Answer from the drawing. Dimensions are ordinates in mm from the lowest x, y and z of the part. Give positions to 0.01 mm unless a question says otherwise; leave off trailing zeros. Loops run counter-clockwise (first coordinate to the right, second up) from the corner with the lowest first, then second, coordinate; pieces in that order, holes last.
Item 1: Section C-C, the plane x = 26 is taken. Give the vertices of the cut face in (y, z) (1 decimal).
Item 2: This flat-tipped pin is pushed along its axis until it touches: pin 1 Ø0.8 at (y, z) = (1.5, 86.5) entering from -X. Where does it stop, or does it pass through?
Item 3: Section B-B, the plane z = 85.5 is taken. Give the vertices of the cut face in (x, y) (1 decimal).
Item 4: Consider line 1 along X through (y, z) = (0.5, 88.5) (1 decimal); line 2 along X through (y, z) = (1, 85) (1 decimal); line 3 along X through (y, z) = (1.95, 67). Determine where each line is inside the solid, lowest interval first.
Item 5: Section A-A, the plane y = 1.9 is taken. Give the vertices of the cut face in (x, z) (1 decimal).
Item 6: Section D-D, the plane z = 65 is taken. Give the vertices of the cut face in (x, y) (1 decimal).
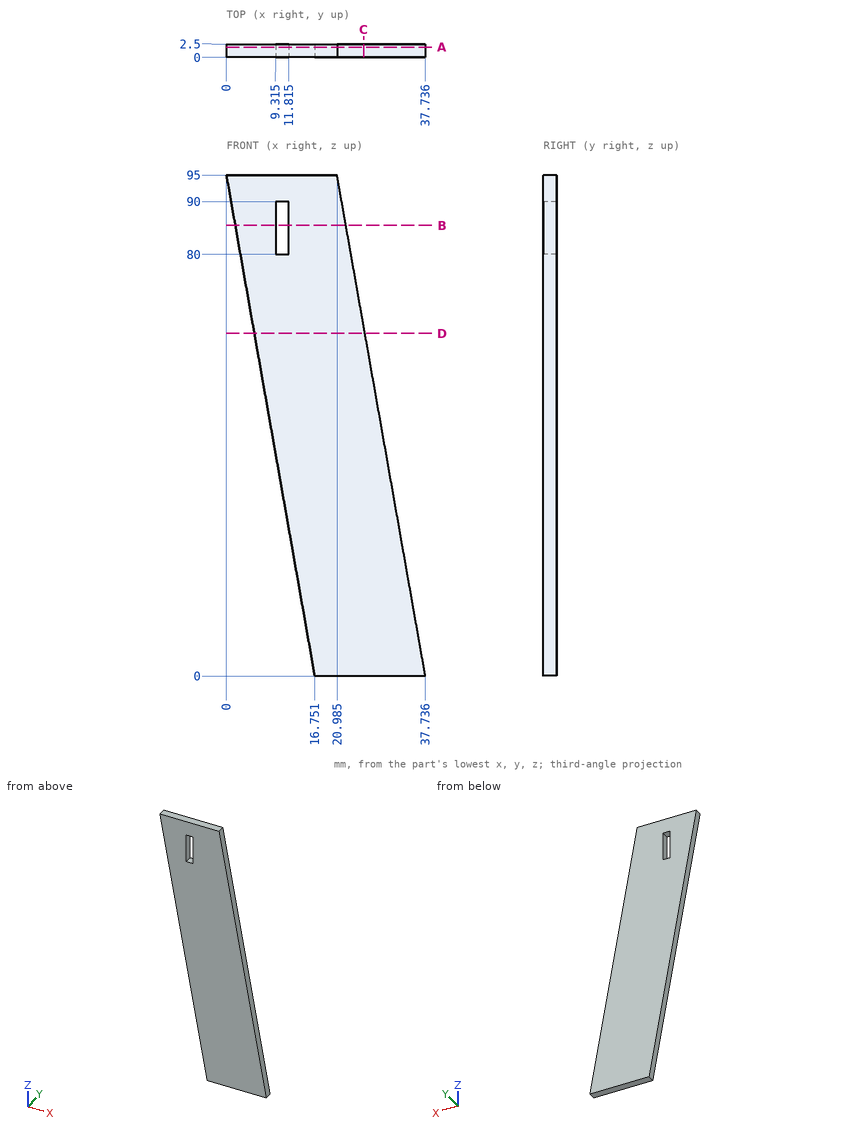
Worked answers:
1. outline: (0, 0) - (2.5, 0) - (2.5, 66.6) - (0, 66.6) - close
2. pin 1: stops at x = 1.43
3. outline: (1.7, 0) - (9.3, 0) - (9.3, 2.5) - (1.7, 2.5) - close; (11.8, 0) - (22.7, 0) - (22.7, 2.5) - (11.8, 2.5) - close
4. line 1: x = 1.1 to 9.3, 11.8 to 22.1
4. line 2: x = 1.8 to 9.3, 11.8 to 22.7
4. line 3: x = 4.94 to 25.92
5. outline: (0, 95) - (16.8, 0) - (37.7, 0) - (21, 95) - close; hole (9.3, 80) - (11.8, 80) - (11.8, 90) - (9.3, 90) - close
6. outline: (5.3, 0) - (26.3, 0) - (26.3, 2.5) - (5.3, 2.5) - close
